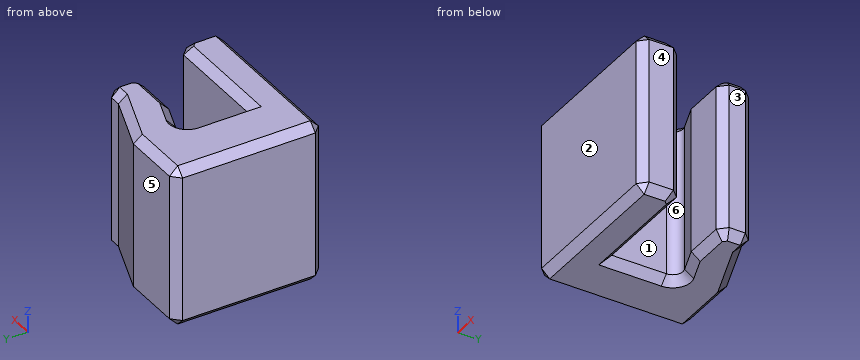
```python
from build123d import *

# Parameters (mm, degrees)
BOSS_EXTRUDE1_DEPTH = 20
CHAMFER1_SIZE       = 1
CHAMFER2_SIZE       = 1


with BuildPart() as part:
    # Sketch1 → Boss-Extrude1 (new body)
    with BuildSketch(Plane.XY):
        with BuildLine():
            Line((0, 6.75), (0, 0))
            Line((0, 0), (14, 0))
            Line((14, 0), (14, -5))
            Line((14, -5), (-7, -5))
            Line((-7, -5), (-7, 13.426942406))
            Line((-7, 13.426942406), (1.274273509, 13.426942406))
            Line((1.274273509, 13.426942406), (8.629112323, 10.75))
            Line((8.629112323, 10.75), (11, 10.75))
            Line((11, 10.75), (11, 6.75))
            Line((11, 6.75), (5, 6.75))
            Line((5, 6.75), (1.710100717, 7.947425413))
            ThreePointArc((1.710100717, 7.947425413), (0.543380251, 7.79382375), (0, 6.75))
        make_face()
    extrude(amount=BOSS_EXTRUDE1_DEPTH)

    # Chamfer1
    chamfer1_edges = [part.edges().sort_by_distance(p)[0] for p in [
        (14, 0, 10),
        (11, 6.75, 10),
    ]]
    chamfer(chamfer1_edges, length=CHAMFER1_SIZE)

    # Chamfer2
    chamfer2_edges = [part.edges().sort_by_distance(p)[0] for p in [
        (6.5, 0, 0),
        (3.355050358, 7.348712706, 20),
        (3.5, -5, 0),
        (-7, 4.213471203, 0),
        (-2.862863246, 13.426942406, 0),
        (4.951692916, 12.088471203, 0),
        (9.814556161, 10.75, 0),
        (11, 9.25, 0),
        (3.355050358, 7.348712706, 0),
        (0.543380251, 7.79382375, 0),
        (0, 3.375, 0),
        (11, 9.25, 20),
        (14, -5, 10),
        (-7, -5, 10),
        (-7, 13.426942406, 10),
        (11, 10.75, 10),
        (9.814556161, 10.75, 20),
        (4.951692916, 12.088471203, 20),
        (-2.862863246, 13.426942406, 20),
        (-7, 4.213471203, 20),
        (14, -3, 0),
        (7.5, 6.75, 0),
        (10.5, 7.25, 0),
        (13.5, -0.5, 0),
        (14, -3, 20),
        (7.5, 6.75, 20),
        (10.5, 7.25, 20),
        (3.5, -5, 20),
        (13.5, -0.5, 20),
        (6.5, 0, 20),
        (0, 3.375, 20),
        (0.543380251, 7.79382375, 20),
    ]]
    chamfer(chamfer2_edges, length=CHAMFER2_SIZE)


solid = part.part
```
Model file for the job. Use its own axes, mm. Face numbers are marked on the shaded views. A direction names the side the tool comes from. Coordinates: 2 decimals unless noted, no trailing zeros. Write each loop counter-clockwise with the first axis right and the second up, starting at its lowest first coordinate (ties: lowest second). Pieces come first, ordered by that corner, then holes. Notation, with made-up numbers: (82.25, 2) - (137.25, 2) arc R28 cw to (137.25, 28) - close; hole circle Ø9 at (-25, 20.25). An arc over 180 degrees is marked (long way). Use a Markdown table: item, result. Add a question column.
Item 1: Drill centre lines: line 1 along Y through (x, z) = (8.75, 10.5); line 2 along X through (y, z) = (0.75, 16); line 3 along Y through (x, z) = (11.5, 7.5). Where is each one in solid material? Low to high.
Item 2: Band-saw the part on D-D, the plane y = -0.5. Write the cut outline in (x, z), and give its area (3 significant figures).
Item 3: Band-saw the part on C-C, the plane z = 2.25. Write the cut outline in (x, y), and give its area (3 significant figures).
Item 4: 3-axis set-ups, long thin cutter, end or side, ignore diameter. For the marked faces 1, 2 and 3: which of +Z, -Z, +X, -X, +Y, -Y reach the whole face in a straight line?
Item 5: Drop flat-ended pins along their axis: pin 1 (1.5 mm diameter, centred on x = 9.5, z = 12, fed in from +Y); pin 2 (3.5 mm diameter, centred on y = 3, z = 8.5, fed in from +X); pin 3 (3 mm diameter, centred on y = 8, z = 10.5, fed in from +X); pin 4 (3 mm diameter, centred on x = 3.5, y = 5.5, fed in from -Z). Give the stop position or say it passes through.
Item 6: Band-saw the part on A-A, the plane y = 5.25. Write the cut outline in (x, z).
Item 7: Two-plate mould, pull along Y, no slides. Class the marked faces 4, 5 and 6: pulls with the +Y half, pulls with the -Y half, needs draft (parallel to the pull), parting line crosses it, or undercut.
Item 8: Band-saw the part on B-B, the plane x = 6.75. Write the cut outline in (y, z).
A:
| question | item | result |
|---|---|---|
| 1 | line 1 | y = -5 to 0, 6.75 to 10.75 |
| 1 | line 2 | x = -7 to 0 |
| 1 | line 3 | y = -5 to 0 |
| 2 | outline | (-7, 1) - (-6, 0) - (-1, 0) - (-0.5, 0.5) - (12.79, 0.5) - (13.5, 1) - (13.5, 19) - (12.79, 19.5) - (-0.5, 19.5) - (-1, 20) - (-6, 20) - (-7, 19) - close |
| 2 | area | 394 mm² |
| 3 | outline | (-7, -4) - (-6, -5) - (13, -5) - (14, -4) - (14, -1) - (13, 0) - (0, 0) - (0, 6.75) arc R1.27 cw to (1.71, 7.95) - (5, 6.75) - (10, 6.75) - (11, 7.75) - (11, 9.75) - (10, 10.75) - (8.63, 10.75) - (1.27, 13.43) - (-6, 13.43) - (-7, 12.43) - close |
| 3 | area | 249 mm² |
| 4 | face 1 | +Z, -Z, +X |
| 4 | face 2 | +Z, -Z, +X, -X, -Y |
| 4 | face 3 | +Z, -Z, +X, +Y |
| 5 | pin 1 | stops at y = 10.75 |
| 5 | pin 2 | stops at x = 0 |
| 5 | pin 3 | stops at x = 11 |
| 5 | pin 4 | passes through |
| 6 | outline | (-7, 1) - (-6, 0) - (-1, 0) - (0, 1) - (0, 19) - (-1, 20) - (-6, 20) - (-7, 19) - close |
| 7 | face 4 | needs draft |
| 7 | face 5 | pulls with the +Y half |
| 7 | face 6 | undercut |
| 8 | outline | (-5, 1) - (-4, 0) - (-1, 0) - (0, 1) - (0, 19) - (-1, 20) - (-4, 20) - (-5, 19) - close; (6.75, 1) - (7.75, 0) - (10.37, 0) - (11.43, 1) - (11.43, 19) - (10.37, 20) - (7.75, 20) - (6.75, 19) - close |
